Geometry check sheet. Reference: the model listing, model coordinates, mm. Round coordinates to 2 decimals unless told otherwise and drop trailing zeros. Write each loop counter-clockwise with the first axis right and the second up, starting at its lowest first coordinate (ties: lowest second). Pieces come first, ordered by that corner, then holes. Notation, with made-up numbers: (38, -16.75) -> (69, -16.75) arc R35 ccw to (69, 18.25) -> close; hole circle Ø8 at (71.5, 84.5). An arc over 180 degrees is marked (long way). Use a Markdown table: item, result.
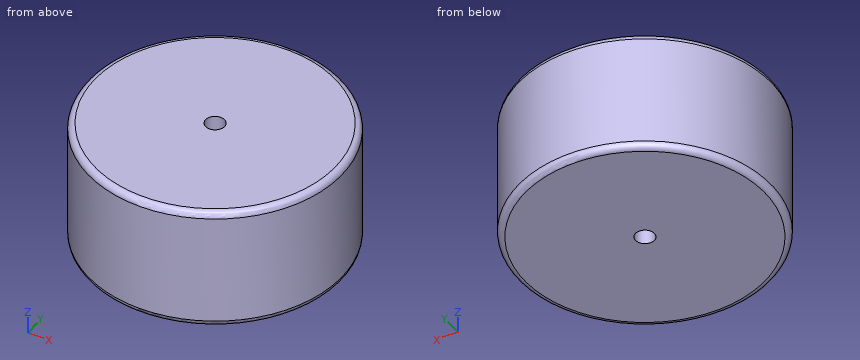
```python
from build123d import *

# Parameters (mm, degrees)
SKETCH_1_R          = 20
EXTRUDE_1_DEPTH     = 19.5
FILLET_1_R          = 1
SKETCH_2_R          = 1.5
CUT_EXTRUDE_1_DEPTH = 20


with BuildPart() as part:
    # 草图1 → 凸台-拉伸1 (new body)
    with BuildSketch(Plane.XY):
        Circle(SKETCH_1_R)
    extrude(amount=EXTRUDE_1_DEPTH)

    # 圆角1
    fillet_1_edges = [part.edges().sort_by_distance(p)[0] for p in [
        (-20, 0, 0),
        (-20, 0, 19.5),
    ]]
    fillet(fillet_1_edges, radius=FILLET_1_R)

    # 草图2 → 切除-拉伸1 (cut)
    with BuildSketch(Plane.XY.offset(19.5)):
        Circle(SKETCH_2_R)
    extrude(amount=-CUT_EXTRUDE_1_DEPTH, mode=Mode.SUBTRACT)


solid = part.part
```
(1) Section check C-C on z = 7.5. Record the cut outline in (x, y).
A:
| item | result |
|---|---|
| outline | circle Ø40 at (0, 0); hole circle Ø3 at (0, 0) |
(2) Section check A-A on y = 0. Record the cut outline in (x, z), plus the area to 3 significant figures.
A:
| item | result |
|---|---|
| outline | (-20, 1) arc R1 ccw to (-19, 0) -> (-1.5, 0) -> (-1.5, 19.5) -> (-19, 19.5) arc R1 ccw to (-20, 18.5) -> close; (1.5, 0) -> (19, 0) arc R1 ccw to (20, 1) -> (20, 18.5) arc R1 ccw to (19, 19.5) -> (1.5, 19.5) -> close |
| area | 721 mm2 |
(3) Gauge pin test, flat ends, axial feed: pin 1 Ø1.5 at (x, z) = (9, 11) entering from +Y; pin 2 Ø5 at (x, z) = (-9.5, 2.5) entering from +Y (3 decimals); pin 3 Ø10 at (x, z) = (4, 15.5) entering from -Y; pin 4 Ø2.5 at (x, y) = (0, 0) entering from -Z. Record the tip position at first contact, or that the pin passes through.
A:
| item | result |
|---|---|
| pin 1 | stops at y = 18.22 |
| pin 2 | stops at y = 18.735 |
| pin 3 | stops at y = -20 |
| pin 4 | passes through |
(4) Thickness scan on line 1 (Y direction, x = 0, z = 15); line 2 (X direction, y = -0.5, z = 17.25); line 3 (Z direction, x = -14, y = 13). Record the ranges inside material, lowest first.
A:
| item | result |
|---|---|
| line 1 | y = -20 to -1.5, 1.5 to 20 |
| line 2 | x = -19.99 to -1.41, 1.41 to 19.99 |
| line 3 | z = 0.01 to 19.49 |
